The model under review builds one solid part; all positions refer to its coordinate system, in mm. A direction names the side the tool comes from. Give positions to 0.01 mm unless a question says otherwise; leave off trailing zeros. Loops run counter-clockwise (first coordinate to the right, second up) from the corner with the lowest first, then second, coordinate; pieces in that order, holes last. Notation, with made-up numbers: M 76.25,52 L 93.25,52 A15 cw 93.25,68 Z; hole C 81.25,49.25 d9. An arc over 180 degrees is marked long. Return JSON: item names as keys, results as strings.
```python
from build123d import *

# Parameters (mm, degrees)
SKETCH_1_R      = 11.1125
SKETCH_1_R_2    = 3.084022448
EXTRUDE_1_DEPTH = 88.9


with BuildPart() as part:
    # Эскиз1 → Бобышка-Вытянуть1 (new body)
    with BuildSketch(Plane(origin=(0, 0, 0), x_dir=(1, 0, 0), z_dir=(0, 1, 0))):
        with BuildLine():
            Line((73.439254163, -13.186564551), (23.385335282, -13.186564551))
            ThreePointArc((23.385335282, -13.186564551), (0, -24.299064551), (-23.385335282, -13.186564551))
            Line((-23.385335282, -13.186564551), (-73.439254163, -13.186564551))
            ThreePointArc((-73.439254163, -13.186564551), (-75.8698, 5.863435449), (-73.439254163, 24.913435449))
            Line((-73.439254163, 24.913435449), (-23.385335282, 24.913435449))
            ThreePointArc((-23.385335282, 24.913435449), (0, 36.025935449), (23.385335282, 24.913435449))
            Line((23.385335282, 24.913435449), (73.439254163, 24.913435449))
            ThreePointArc((73.439254163, 24.913435449), (75.8698, 5.863435449), (73.439254163, -13.186564551))
        make_face()
        with Locations(Location((0, 5.863435449, 0), (0, 0, 270))):
            Circle(SKETCH_1_R, mode=Mode.SUBTRACT)
        with Locations(Location((-57.15, 5.863435449, 0), (0, 0, 270))):
            Circle(SKETCH_1_R_2, mode=Mode.SUBTRACT)
        with Locations(Location((57.15, 5.863435449, 0), (0, 0, 90))):
            Circle(SKETCH_1_R_2, mode=Mode.SUBTRACT)
    extrude(amount=EXTRUDE_1_DEPTH)


solid = part.part
```
1) Insertion check: pin 1 (3.5 mm diameter, centred on x = 57.15, z = -5.86, fed in from +Y); pin 2 (15 mm diameter, centred on x = -37.5, y = 44.5, fed in from +Z); pin 3 (8 mm diameter, centred on x = -53.5, y = 47, fed in from -Z); pin 4 (12 mm diameter, centred on x = -22.5, y = 53.5, fed in from +Z). Each pin has a flat end and moves straight along its axis. Give the tip position at first contact, or say it passes through.
From the geometry:
{"pin 1": "through", "pin 2": "z = 13.19", "pin 3": "z = -24.91", "pin 4": "z = 19.39"}
2) Tool access review of faces 4 (the face through (48, 44, -24.913)), 5 (the face through (49, 44, 13.187)), 6 (the face through (-49, 44, -24.913)), 7 (the face through (-48, 44, 13.187)): name each direction out of +Z, -Z, +X, -X, +Y, -Y from which nothing blocks a thin tool from reaching the whole face with its end or side.
From the geometry:
{"face 4": "-Z, +X, +Y, -Y", "face 5": "+Z, +X, +Y, -Y", "face 6": "-Z, -X, +Y, -Y", "face 7": "+Z, -X, +Y, -Y"}
3) Consider section A-A on x = 57.15. Write out the cut boundary in (y, z).
From the geometry:
{"outline": "M 0,-24.91 L 88.9,-24.91 L 88.9,-8.95 L 0,-8.95 Z; M 0,-2.78 L 88.9,-2.78 L 88.9,13.19 L 0,13.19 Z"}
4) Consider section B-B on y = 24. Count the separate pieces of the cut face and the enclosed holes in it, then the cut area to 3 significant figures.
From the geometry:
{"separate pieces": "1", "enclosed holes": "3", "area": "6,000 mm²"}
5) Wall thickness on L1, parallel to X at y = 74.5, z = -6; L2, parallel to Z at x = 57.15, y = 50.5; L3, parallel to Z at x = 0.5, y = 77: over which ranges is each line inside the solid? List them lowest first. Write a range as from..to.
From the geometry:
{"L1": "-75.87..-60.23, -54.07..-11.11, 11.11..54.07, 60.23..75.87", "L2": "-24.91..-8.95, -2.78..13.19", "L3": "-36.02..-16.96, 5.24..24.29"}
6) The part is to be moulded in two halves that separate along Z. For faces 1 (the face through (75.87, 43.83, -6.13)), 2 (the face through (-0.375, 43.828, -36.024)), 3 (the face through (59.886, 43.828, -7.287)), say which applies: released by +Z, released by -Z, zero draft, split by the parting line, or undercut.
From the geometry:
{"face 1": "split by the parting line", "face 2": "released by -Z", "face 3": "undercut"}
7) Consider section C-C on z = -5. Write out the cut boundary in (x, y), then the cut area to 3 significant figures.
From the geometry:
{"outline": "M -75.86,0 L -60.11,0 L -60.11,88.9 L -75.86,88.9 Z; M -54.19,0 L -11.08,0 L -11.08,88.9 L -54.19,88.9 Z; M 11.08,0 L 54.19,0 L 54.19,88.9 L 11.08,88.9 Z; M 60.11,0 L 75.86,0 L 75.86,88.9 L 60.11,88.9 Z", "area": "10,500 mm²"}
8) Consider section D-D on z = -13. Write out the cut boundary in (x, y), then the cut area to 3 significant figures.
From the geometry:
{"outline": "M -75.53,0 L -8.52,0 L -8.52,88.9 L -75.53,88.9 Z; M 8.52,0 L 75.53,0 L 75.53,88.9 L 8.52,88.9 Z", "area": "11,900 mm²"}
